Geometry check sheet. Reference: the model listing, model coordinates, mm. A direction names the side the tool comes from. Coordinates: 2 decimals unless noted, no trailing zeros. Write each loop counter-clockwise with the first axis right and the second up, starting at its lowest first coordinate (ties: lowest second). Pieces come first, ordered by that corner, then holes.
from build123d import *

# Parameters (mm, degrees)
SKETCH_1_W          = 26
SKETCH_1_H          = 38
EXTRUDE_1_DEPTH     = 10
SKETCH_2_W          = 22
SKETCH_2_H          = 34
CUT_EXTRUDE_1_DEPTH = 8
SKETCH_4_W          = 6
SKETCH_4_H          = 6
EXTRUDE_2_DEPTH     = 3
SKETCH_5_R          = 1
CUT_EXTRUDE_4_DEPTH = 11
FILLET_1_R          = 5


with BuildPart() as part:
    # ｽｹｯﾁ1 → ﾎﾞｽ - 押し出し1 (new body)
    with BuildSketch(Plane.XY):
        Rectangle(SKETCH_1_W, SKETCH_1_H)
    extrude(amount=EXTRUDE_1_DEPTH)

    # ｽｹｯﾁ2 → ｶｯﾄ - 押し出し1 (cut)
    with BuildSketch(Plane.XY):
        Rectangle(SKETCH_2_W, SKETCH_2_H)
    extrude(amount=CUT_EXTRUDE_1_DEPTH, mode=Mode.SUBTRACT)

    # ｽｹｯﾁ4 → ﾎﾞｽ - 押し出し2 (add)
    with BuildSketch(Plane.XY):
        with Locations((16, 16)):
            Rectangle(SKETCH_4_W, SKETCH_4_H)
        with Locations((16, -16)):
            Rectangle(SKETCH_4_W, SKETCH_4_H)
        with Locations((-16, -16)):
            Rectangle(SKETCH_4_W, SKETCH_4_H)
        with Locations((-16, 16)):
            Rectangle(SKETCH_4_W, SKETCH_4_H)
    extrude(amount=EXTRUDE_2_DEPTH)

    # ｽｹｯﾁ5 → ｶｯﾄ - 押し出し4 (cut, through all)
    with BuildSketch(Plane.XY):
        with Locations((-16, 16)):
            Circle(SKETCH_5_R)
        with Locations((-16, -16)):
            Circle(SKETCH_5_R)
        with Locations((16, -16)):
            Circle(SKETCH_5_R)
        with Locations((16, 16)):
            Circle(SKETCH_5_R)
    extrude(amount=CUT_EXTRUDE_4_DEPTH, mode=Mode.SUBTRACT)

    # ﾌｨﾚｯﾄ1
    fillet_1_edges = [part.edges().sort_by_distance(p)[0] for p in [
        (0, 19, 10),
        (0, -19, 10),
        (13, 0, 10),
        (-13, 0, 10),
    ]]
    fillet(fillet_1_edges, radius=FILLET_1_R)


solid = part.part
1. Draft check along Y on faces 1 (the flat face through (16, 13, 1)), 2 (the flat face through (-11, 0, 4)), 3 (the flat face through (-19, 16, 1)), 4 (the flat face through (0, 19, 2)). Enter one of: released by +Y, released by -Y, zero draft, split by the parting line, or undercut.
Computed values:
face 1: undercut
face 2: undercut
face 3: zero draft
face 4: released by +Y
2. Sectioned sample at A-A, the plane x = -16. Record the boundary of the cut face in (y, z), and give its area (3 significant figures).
Computed values:
outline: (-19, 0) - (-17, 0) - (-17, 3) - (-19, 3) - close; (-15, 0) - (-13, 0) - (-13, 3) - (-15, 3) - close; (13, 0) - (15, 0) - (15, 3) - (13, 3) - close; (17, 0) - (19, 0) - (19, 3) - (17, 3) - close
area: 24.0 mm2
3. Sectioned sample at D-D, the plane y = 11.5. Record the boundary of the cut face in (x, z).
Computed values:
outline: (-13, 0) - (-11, 0) - (-11, 8) - (11, 8) - (11, 0) - (13, 0) - (13, 5) arc R5 ccw to (8, 10) - (-8, 10) arc R5 ccw to (-13, 5) - close
4. Thickness scan on line 1 along Y through (x, z) = (16, 1.85); line 2 along X through (y, z) = (-16, 1.5); line 3 along Y through (x, z) = (7, 1.5). Record the ranges inside material, lowest first.
Computed values:
line 1: y = -19 to -17, -15 to -13, 13 to 15, 17 to 19
line 2: x = -19 to -17, -15 to -11, 11 to 15, 17 to 19
line 3: y = -19 to -17, 17 to 19
5. Access from +Z, -Z, +X, -X, +Y, -Y to the whole of each face (thin tool, end or side, straight path). Record for faces 5 (the flat face through (0, 17, 4)), 6 (the flat face through (16, -13, 1)), 7 (the flat face through (-17, 17, 3)), 8 (the flat face through (15, 17, 3)).
Computed values:
face 5: -Z
face 6: +Z, -Z, +X
face 7: +Z, -X, +Y, -Y
face 8: +Z, +X, +Y, -Y
6. Sectioned sample at B-B, the plane z = 2.5. Record the boundary of the cut face in (x, y), and give its area (3 significant figures).
Computed values:
outline: (-19, -19) - (19, -19) - (19, -13) - (13, -13) - (13, 13) - (19, 13) - (19, 19) - (-19, 19) - (-19, 13) - (-13, 13) - (-13, -13) - (-19, -13) - close; hole circle Ø2 at (-16, -16); hole circle Ø2 at (-16, 16); hole (-11, -17) - (11, -17) - (11, 17) - (-11, 17) - close; hole circle Ø2 at (16, -16); hole circle Ø2 at (16, 16)
area: 371 mm2
7. Sectioned sample at C-C, the plane y = -16. Record the boundary of the cut face in (x, z), and give its area (3 significant figures).
Computed values:
outline: (-19, 0) - (-17, 0) - (-17, 3) - (-19, 3) - close; (-15, 0) - (-11, 0) - (-11, 8) - (11, 8) - (11, 0) - (15, 0) - (15, 3) - (13, 3) - (13, 5) arc R5 ccw to (10, 9.58) - (-10, 9.58) arc R5 ccw to (-13, 5) - (-13, 3) - (-15, 3) - close; (17, 0) - (19, 0) - (19, 3) - (17, 3) - close
area: 89.5 mm2
8. Gauge pin test, flat ends, axial feed: pin 1 Ø1 at (x, y) = (-0.5, 0.5) entering from -Z; pin 2 Ø3 at (x, y) = (16.5, -17) entering from +Z; pin 3 Ø2 at (y, z) = (-13, 7) entering from +X. Record the tip position at first contact, or that the pin passes through.
Computed values:
pin 1: stops at z = 8
pin 2: stops at z = 3
pin 3: stops at x = 12.9
